CAD build for the part. Positions are in the model's coordinates, mm. Face numbers are marked on the shaded views. Give positions to 0.01 mm unless a question says otherwise; leave off trailing zeros. Write item = value, one per line. Start each with the question number.
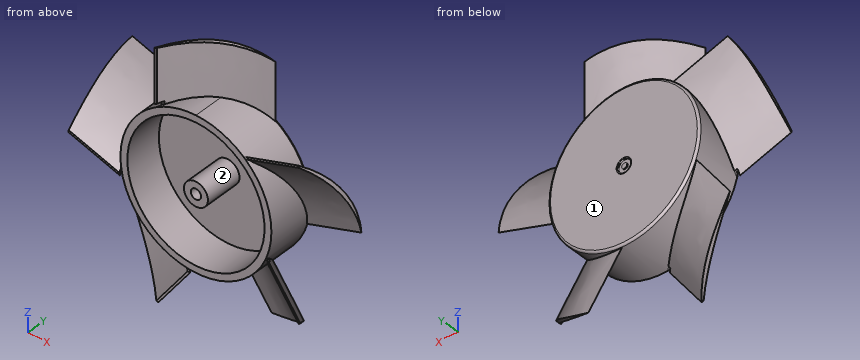
```python
from build123d import *

# Parameters (mm, degrees)
SKETCH1_R                = 11
BOSS_EXTRUDE1_DEPTH      = 7
BOSS_EXTRUDE2_REACH      = 19.059
BOSS_EXTRUDE2_END_RADIUS = 18.55
CIRPATTERN1_COUNT        = 5
SKETCH4_R                = 10
SKETCH4_R_2              = 1.75
SKETCH4_R_3              = 0.75
CUT_EXTRUDE1_DEPTH       = 5.5
FILLET1_R                = 0.3
SKETCH5_R                = 1
CUT_EXTRUDE2_DEPTH       = 0.2
FILLET2_R                = 0.1
SKETCH6_R                = 11.4
SKETCH6_R_2              = 11
CUT_EXTRUDE3_DEPTH       = 0.6
SKETCH7_R                = 0.4
BOSS_EXTRUDE3_DEPTH      = 0.1


with BuildPart() as part:
    # Sketch1 → Boss-Extrude1 (new body)
    with BuildSketch(Plane(origin=(0, 0, 0), x_dir=(1, 0, 0), z_dir=(0, 1, 0))):
        with Locations(Location((0, 0, 0), (0, 0, 270))):
            Circle(SKETCH1_R)
    extrude(amount=BOSS_EXTRUDE1_DEPTH)

    # Boss-Extrude2: up to this cylinder (the profile starts inside it)
    boss_extrude2_end = Plane(origin=(0, 3.843243, 0), z_dir=(0, -1, 0)) * Cylinder(BOSS_EXTRUDE2_END_RADIUS, 76.218, mode=Mode.PRIVATE)
    # Sketch2 → Boss-Extrude2 (add, up to the surface)
    with BuildSketch(Plane.XY, mode=Mode.PRIVATE) as boss_extrude2_sk1:
        with BuildLine():
            Line((-6, 0), (-5.7, 0))
            add(Edge.make_bspline(
                [(6, 6.65), (-0.86634689, 4.993225635), (-5.7, 0)],
                knots=[0, 0, 0, 1, 1, 1], degree=2))
            add(Edge.make_bspline(
                [(6, 6.65), (-1.357374642, 5.918314261), (-6, 0)],
                knots=[0, 0, 0, 1, 1, 1], degree=2))
        make_face()
    boss_extrude2_tool1 = extrude(boss_extrude2_sk1.sketch, amount=BOSS_EXTRUDE2_REACH, mode=Mode.PRIVATE) & boss_extrude2_end
    boss_extrude2 = boss_extrude2_tool1.solids().sort_by_distance((-0.900536, 3.843243, 0))[0]
    add(boss_extrude2)

    # CirPattern1: Boss-Extrude2 ×5 about axis
    cirpattern1_axis = Axis((0, 7, 0), (0, -1, 0))
    for i in range(1, CIRPATTERN1_COUNT):
        add(boss_extrude2.rotate(cirpattern1_axis, i * 360 / CIRPATTERN1_COUNT))

    # Sketch4 → Cut-Extrude1 (cut)
    # profile 1 of 2: a face of its own
    with BuildSketch(Plane.XZ):
        with Locations(Location((0, 0, 0), (0, 0, 270))):
            Circle(SKETCH4_R)
        with Locations(Location((0, 0, 0), (0, 0, 270))):
            Circle(SKETCH4_R_2, mode=Mode.SUBTRACT)
    # profile 2 of 2: a face of its own
    with BuildSketch(Plane.XZ):
        with Locations(Location((0, 0, 0), (0, 0, 270))):
            Circle(SKETCH4_R_3)
    extrude(amount=-CUT_EXTRUDE1_DEPTH, mode=Mode.SUBTRACT)

    # Fillet1
    fillet1_edges = [part.edges().sort_by_distance(p)[0] for p in [
        (0, 7, -11),
    ]]
    fillet(fillet1_edges, radius=FILLET1_R)

    # Sketch5 → Cut-Extrude2 (cut)
    with BuildSketch(Plane(origin=(0, 7, 0), x_dir=(1, 0, 0), z_dir=(0, 1, 0))):
        with Locations(Location((0, 0, 0), (0, 0, 270))):
            Circle(SKETCH5_R)
    extrude(amount=-CUT_EXTRUDE2_DEPTH, mode=Mode.SUBTRACT)

    # Fillet2
    fillet2_edges = [part.edges().sort_by_distance(p)[0] for p in [
        (0, 6.8, -1),
        (0, 7, -1),
    ]]
    fillet(fillet2_edges, radius=FILLET2_R - 0.0001)  # a hair under: the kernel refuses the full size

    # Sketch6 → Cut-Extrude3 (cut)
    with BuildSketch(Plane.XZ):
        Circle(SKETCH6_R)
        with Locations(Location((0, 0, 0), (0, 0, 90))):
            Circle(SKETCH6_R_2, mode=Mode.SUBTRACT)
    extrude(amount=-CUT_EXTRUDE3_DEPTH, mode=Mode.SUBTRACT)

    # Sketch7 → Boss-Extrude3 (add)
    with BuildSketch(Plane(origin=(0, 6.8, 0), x_dir=(1, 0, 0), z_dir=(0, 1, 0))):
        with Locations(Location((0, 0, 0), (0, 0, 270))):
            Circle(SKETCH7_R)
    extrude(amount=BOSS_EXTRUDE3_DEPTH)


solid = part.part
```
1. Wall check: line 1 along X through (y, z) = (3.6, 0); line 2 along Z through (x, y) = (-8.5, 3); line 3 along Z through (x, y) = (1, 3). Give the ranges that are in metal, low to high.
2. Cut at A-A (y = 3.5). Count the separate pieces of the cut face and the enclosed holes in it, then the cut area to 3 significant figures.
3. Mould opens along Z. For the marked faces 1 and 2 say: +Z half, -Z half, draft (parallel to the pull), parting line (faces both ways), or undercut.
4. Pin check, flat tips, straight feed: pin 1 Ø10 at (x, z) = (-3.5, 4.5) entering from -Y; pin 2 Ø1.5 at (x, z) = (3.5, -12.5) entering from -Y; pin 3 Ø2 at (x, z) = (1.5, -7) entering from -Y; pin 4 Ø1.5 at (y, z) = (2, 1) entering from +X. Stop position of each tip, or through.
Output:
q1.line_1 = -11 to -10, -1.75 to -0.75, 0.75 to 1.75, 10 to 11
q1.line_2 = -16.49 to -15.43, -6.98 to -5.27, 5.27 to 6.98
q1.line_3 = -10.95 to -9.95, -1.44 to 1.44, 9.95 to 10.95
q2.separate_pieces = 2
q2.enclosed_holes = 2
q2.area = 111 mm2
q3.face_1 = draft
q3.face_2 = undercut
q4.pin_1 = 0
q4.pin_2 = 6
q4.pin_3 = 5.5
q4.pin_4 = 11
